from build123d import *

# Parameters (mm, degrees)
SKETCH1_R           = 2.5
BOSS_EXTRUDE1_DEPTH = 3
SKETCH2_R           = 3.464101615
SKETCH2_R_2         = 2.5
BOSS_EXTRUDE2_DEPTH = 2
FILLET1_R           = 0.1


with BuildPart() as part:
    # Sketch1 → Boss-Extrude1 (new body)
    with BuildSketch(Plane(origin=(0, 0, 0), x_dir=(1, 0, 0), z_dir=(0, 1, 0))):
        Polygon((0, 4), (-3.464101615, 2), (-3.464101615, -2), (0, -4), (3.464101615, -2), (3.464101615, 2), align=None)
        with Locations(Location((0, 0, 0), (0, 0, 270))):
            Circle(SKETCH1_R, mode=Mode.SUBTRACT)
    extrude(amount=BOSS_EXTRUDE1_DEPTH)

    # Sketch2 → Boss-Extrude2 (add)
    with BuildSketch(Plane(origin=(0, 3, 0), x_dir=(1, 0, 0), z_dir=(0, 1, 0))):
        with Locations(Location((0, 0, 0), (0, 0, 60))):
            Circle(SKETCH2_R)
        with Locations(Location((0, 0, 0), (0, 0, 270))):
            Circle(SKETCH2_R_2, mode=Mode.SUBTRACT)
    extrude(amount=BOSS_EXTRUDE2_DEPTH)

    # Fillet1
    fillet1_edges = [part.edges().sort_by_distance(p)[0] for p in [
        (-1.732050808, 5, 3),
    ]]
    fillet(fillet1_edges, radius=FILLET1_R)


solid = part.part
Verification items for the finished model (mm, model axes). A direction names the side the tool comes from. Give positions to 0.01 mm unless a question says otherwise; leave off trailing zeros. Loops run counter-clockwise (first coordinate to the right, second up) from the corner with the lowest first, then second, coordinate; pieces in that order, holes last.
1. Cross-section at A-A on y = 1.95. Record the cut outline in (x, z).
Derived:
outline: (-3.46, -2) - (0, -4) - (3.46, -2) - (3.46, 2) - (0, 4) - (-3.46, 2) - close; hole circle Ø5 at (0, 0)
2. Material ranges on probe 1 along X at (y, z) = (2.35, 0); probe 2 along X at (y, z) = (2.85, 1.5); probe 3 along Z at (x, y) = (-1.75, 4.05), recorded low to high.
Derived:
probe 1: x = -3.46 to -2.5, 2.5 to 3.46
probe 2: x = -3.46 to -2, 2 to 3.46
probe 3: z = -2.99 to -1.79, 1.79 to 2.99
3. Go/stop test with flat-tipped pins: P1, Ø0.8, axis at x = 1, z = -3.5, coming from the +Y side; P2, Ø1.5, axis at x = -1.5, z = 0.5, coming from the -Y side. Record where each tip stops, or that it passes through.
Derived:
P1: stops at y = 5
P2: passes through
4. Tool access check on faces 1 (the flat face through (3.2, 3, -1.7)), 2 (the flat face through (-0.01, 3, 3.65)), 3 (the flat face through (-3.12, 3, -1.84)), 4 (the flat face through (-3.12, 3, 1.83)). Record the directions out of +Z, -Z, +X, -X, +Y, -Y that give a thin tool (end or side, any length) a straight path to the whole face; none if there is none.
Derived:
face 1: -Z, +X, +Y
face 2: +Z, +Y
face 3: -Z, -X, +Y
face 4: +Z, -X, +Y
5. Cross-section at B-B on y = 4.45. Record the cut outline in (x, z), and give its area (3 significant figures).
Derived:
outline: circle Ø6.93 at (0, 0); hole circle Ø5 at (0, 0)
area: 18.1 mm2
6. Release check for a two-part mould opening along Z. For faces 5 (the flat face through (1.708, 1.479, 3.014)), 6 (the cylindrical face through (-3.2, 3.94, -1.33)), 7 (the cylindrical face through (-2.44, 2.46, -0.54)), 8 (the flat face through (0, 0, 3)) record: +Z half, -Z half, draft (parallel to the pull), parting line (faces both ways), or undercut.
Derived:
face 5: +Z half
face 6: parting line
face 7: undercut
face 8: draft
